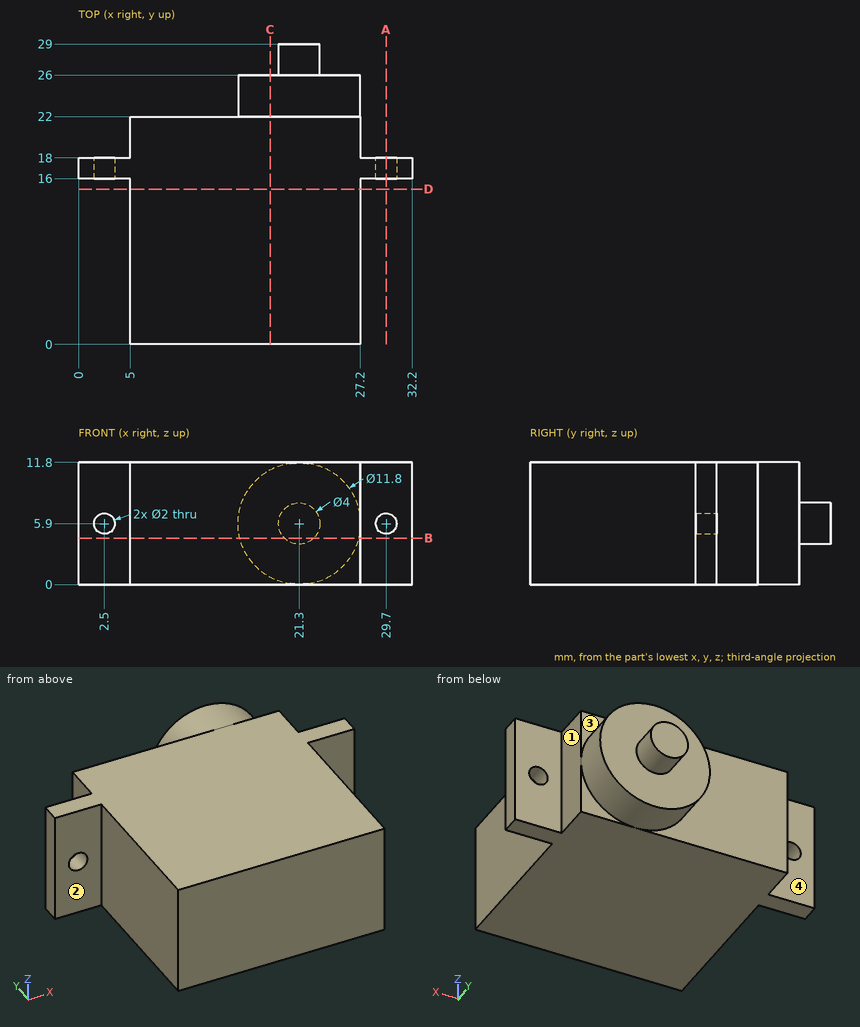
Could you check a few things on this drawing? It's one solid part, dimensions in mm from its lowest x, y, z. A direction names the side the tool comes from. Round coordinates to 2 decimals unless told otherwise and drop trailing zeros. Write each loop counter-clockwise with the first axis right and the second up, starting at its lowest first coordinate (ties: lowest second). Pieces come first, ordered by that corner, then holes.
Q1. If we section it at D-D on y = 15: Write out the boundary of the cut face in (x, z), plus the area to 3 significant figures.
Q2. If we section it at C-C on x = 18.5: Write out the boundary of the cut face in (y, z), plus the area to 3 significant figures.
Q3. Will these pins go through, and if not, where does the flat tip stop? P1, Ø3, axis at y = 8, z = 9.5, coming from the +X side; P2, Ø2.5, axis at x = 3, z = 4.5, coming from the -Y side; P3, Ø1.5, axis at x = 31, z = 7.5, coming from the +Y side.
Q4. If we section it at A-A on x = 29.7: Write out the boundary of the cut face in (y, z), plus the area to 3 significant figures.
Q5. Which directions (+Z, -Z, +X, -X, +Y, -Y) give clear straight access to the entire face, cutting with the end or side of a thin tool? Please do the marked faces 1, 2, 3 and 4.
Q6. Please list where these lines run through material, in increasing order: probe 1 along X at (y, z) = (17.3, 5.9); probe 2 along Z at (x, y) = (29.7, 16.65); probe 3 along Y at (x, z) = (22.5, 10).
Q7. If we section it at B-B on z = 4.5: Write out the boundary of the cut face in (x, y).
Answer below:
1. outline: (5, 0) - (27.2, 0) - (27.2, 11.8) - (5, 11.8) - close
1. area: 262 mm2
2. outline: (0, 0) - (22, 0) - (22, 0.71) - (26, 0.71) - (26, 11.09) - (22, 11.09) - (22, 11.8) - (0, 11.8) - close
2. area: 301 mm2
3. P1: stops at x = 27.2
3. P2: stops at y = 16
3. P3: stops at y = 18
4. outline: (16, 0) - (18, 0) - (18, 4.9) - (16, 4.9) - close; (16, 6.9) - (18, 6.9) - (18, 11.8) - (16, 11.8) - close
4. area: 19.6 mm2
5. face 1: +Z, -Z, +X, +Y
5. face 2: +Z, -Z, -X, -Y
5. face 3: +Z, +X, +Y
5. face 4: +Z, -Z, -X, +Y
6. probe 1: x = 0 to 1.5, 3.5 to 28.7, 30.7 to 32.2
6. probe 2: z = 0 to 4.9, 6.9 to 11.8
6. probe 3: y = 0 to 26
7. outline: (0, 16) - (5, 16) - (5, 0) - (27.2, 0) - (27.2, 16) - (32.2, 16) - (32.2, 18) - (27.2, 18) - (27.2, 22) - (27.03, 22) - (27.03, 26) - (22.73, 26) - (22.73, 29) - (19.87, 29) - (19.87, 26) - (15.57, 26) - (15.57, 22) - (5, 22) - (5, 18) - (0, 18) - close
